```python
from build123d import *

# Parameters (mm, degrees)
SKETCH1_W               = 76.708
SKETCH1_H               = 32.2799964
SKETCH1_R               = 3.571875
MAIN_BODY_DEPTH         = 34
SKETCH13_W              = 76.708
SKETCH13_H              = 25.9299964
CUT_EXTRUDE1_DEPTH      = 27.65
SKETCH14_OUTSIDE_W      = 96.688
SKETCH14_OUTSIDE_H      = 52.26
SKETCH14_OUTSIDE_W_2    = 70.612
SKETCH14_OUTSIDE_H_2    = 32.2799964
CUT_EXTRUDE2_DEPTH      = 1
CUT_EXTRUDE2_DEPTH_BACK = 35


with BuildPart() as part:
    # Sketch1 → Main Body (new body)
    with BuildSketch(Plane(origin=(0, 0, 0), x_dir=(1, 0, 0), z_dir=(0, 1, 0))):
        with Locations((38.354, 16.1399982)):
            Rectangle(SKETCH1_W, SKETCH1_H)
        with Locations((19.177, 16.1399982)):
            Circle(SKETCH1_R, mode=Mode.SUBTRACT)
        with Locations((57.531, 16.1399982)):
            Circle(SKETCH1_R, mode=Mode.SUBTRACT)
    extrude(amount=MAIN_BODY_DEPTH)

    # Sketch13 → Cut-Extrude1 (cut)
    with BuildSketch(Plane(origin=(0, 34, 0), x_dir=(1, 0, 0), z_dir=(0, 1, 0))):
        with Locations((38.354, 19.3149982)):
            Rectangle(SKETCH13_W, SKETCH13_H)
    extrude(amount=-CUT_EXTRUDE1_DEPTH, mode=Mode.SUBTRACT)

    # Sketch14 outside → Cut-Extrude2 (cut, two sides)
    with BuildSketch(Plane.XZ) as cut_extrude2_sk:
        with Locations((38.354, -16.14)):
            Rectangle(SKETCH14_OUTSIDE_W, SKETCH14_OUTSIDE_H)
        with Locations((38.354, -16.1399982)):
            Rectangle(SKETCH14_OUTSIDE_W_2, SKETCH14_OUTSIDE_H_2, mode=Mode.SUBTRACT)
    extrude(amount=CUT_EXTRUDE2_DEPTH, mode=Mode.SUBTRACT)
    extrude(cut_extrude2_sk.sketch, amount=-CUT_EXTRUDE2_DEPTH_BACK, mode=Mode.SUBTRACT)


solid = part.part
```
Can you work these out from the model? Positions are in its coordinate system, mm. A direction names the side the tool comes from. Give positions to 0.01 mm unless a question says otherwise; leave off trailing zeros. Write each loop counter-clockwise with the first axis right and the second up, starting at its lowest first coordinate (ties: lowest second). Pieces come first, ordered by that corner, then holes. Notation, with made-up numbers: (71.25, -37) -> (105.25, -37) arc R12 cw to (105.25, -15) -> close; hole circle Ø10 at (33.25, -27). An arc over 180 degrees is marked (long way). Write item = value, one per line.
(1) For faces 1 (the face through (38, 20, -6.35)), 2 (the face through (38, 0, -16)), which set-ups out of +Z, -Z, +X, -X, +Y, -Y let a thin tool reach every point of the face, with its end or its side?
Worked out:
face_1 = -Z, +X, -X, +Y
face_2 = +Z, -Z, +X, -X, -Y
(2) I'm going to push flat-ended pins straight in: P1, Ø10, axis at x = 17, z = -13.5, coming from the +Y side; P2, Ø1.5, axis at x = 38.5, y = 26, coming from the +Z side; P3, Ø6.5, axis at x = 57.53, z = -16.14, coming from the -Y side; P4, Ø2, axis at x = 46.5, y = 10, coming from the -Z side. Where does each tip first touch, or does it pass through?
Worked out:
P1 = 6.35
P2 = 0
P3 = through
P4 = -6.35
(3) Suppose I cut it at A-A on z = -18. Write out the boundary of the cut face in (x, y), then the cut area to 3 significant figures.
Worked out:
outline = (3.05, 0) -> (16.13, 0) -> (16.13, 6.35) -> (3.05, 6.35) -> close; (22.23, 0) -> (54.48, 0) -> (54.48, 6.35) -> (22.23, 6.35) -> close; (60.58, 0) -> (73.66, 0) -> (73.66, 6.35) -> (60.58, 6.35) -> close
area = 371 mm^2
(4) I need wall thicknesses on probe 1 along Y at (x, z) = (15.5, -17.5); probe 2 along Z at (x, y) = (38, 13). Which ranges of each line are inside material? Lowest first, please. Write a range as from..to.
Worked out:
probe_1 = 0..6.35
probe_2 = -6.35..0
(5) Suppose I cut it at C-C on x = 67. Write out the boundary of the cut face in (y, z).
Worked out:
outline = (0, -32.28) -> (6.35, -32.28) -> (6.35, -6.35) -> (34, -6.35) -> (34, 0) -> (0, 0) -> close
(6) Suppose I cut it at B-B on x = 19.5. Write out the boundary of the cut face in (y, z).
Worked out:
outline = (0, -32.28) -> (6.35, -32.28) -> (6.35, -19.7) -> (0, -19.7) -> close; (0, -12.58) -> (6.35, -12.58) -> (6.35, -6.35) -> (34, -6.35) -> (34, 0) -> (0, 0) -> close
(7) Thinking about a two-plate mould opening in X: for faces 3 (the face through (18.403, 3.131, -12.653)), 4 (the face through (73.66, 9, -6)), 5 (the face through (38, 3, -32.28)), which applies, released by +X, released by -X, zero draft, split by the parting line, or undercut?
Worked out:
face_3 = undercut
face_4 = released by +X
face_5 = zero draft
(8) Suppose I cut it at D-D on y = 24. Write out the boundary of the cut face in (x, z), then the cut area to 3 significant figures.
Worked out:
outline = (3.05, -6.35) -> (73.66, -6.35) -> (73.66, 0) -> (3.05, 0) -> close
area = 448 mm^2
